The listing builds one solid part. Answer for the finished solid, in the listing's coordinates (mm). Coordinates: 2 decimals unless noted, no trailing zeros. Loops run counter-clockwise (first coordinate to the right, second up) from the corner with the lowest first, then second, coordinate; pieces in that order, holes last. Notation, with made-up numbers: (10.5, 65) - (37.5, 65) arc R22 ccw to (37.5, 86) - close; hole circle Ø10 at (89, 74). An arc over 180 degrees is marked (long way). Put each result on its own line as item: value.
```python
from build123d import *

# Parameters (mm, degrees)
SKETCH1_W              = 78
SKETCH1_H              = 120
SKETCH1_R              = 1.5
SKETCH1_W_2            = 4
SKETCH1_H_2            = 68
MAIN_SLIDER_TOP_DEPTH  = 2
SLIDE_TOP_CONTOURING_R = 4


with BuildPart() as part:
    # Sketch1 → Main Slider Top (new body)
    with BuildSketch(Plane.XY):
        with Locations((39, 60)):
            Rectangle(SKETCH1_W, SKETCH1_H)
        with Locations((14, 108)):
            Circle(SKETCH1_R, mode=Mode.SUBTRACT)
        with Locations((32, 108)):
            Circle(SKETCH1_R, mode=Mode.SUBTRACT)
        with Locations((14, 24)):
            Circle(SKETCH1_R, mode=Mode.SUBTRACT)
        with Locations((32, 24)):
            Circle(SKETCH1_R, mode=Mode.SUBTRACT)
        with Locations((46, 108)):
            Circle(SKETCH1_R, mode=Mode.SUBTRACT)
        with Locations((64, 108)):
            Circle(SKETCH1_R, mode=Mode.SUBTRACT)
        with Locations((46, 24)):
            Circle(SKETCH1_R, mode=Mode.SUBTRACT)
        with Locations((64, 24)):
            Circle(SKETCH1_R, mode=Mode.SUBTRACT)
        with Locations((23, 73)):
            Rectangle(SKETCH1_W_2, SKETCH1_H_2, mode=Mode.SUBTRACT)
        with Locations((55, 73)):
            Rectangle(SKETCH1_W_2, SKETCH1_H_2, mode=Mode.SUBTRACT)
        with BuildLine():
            Line((32, 118), (32, 116))
            add(Edge.make_bspline(
                [(32, 116), (39, 116.4), (46, 116)],
                knots=[0, 0, 0, 1, 1, 1], degree=2))
            Line((46, 116), (46, 118))
            add(Edge.make_bspline(
                [(32, 118), (39, 117.6), (46, 118)],
                knots=[0, 0, 0, 1, 1, 1], degree=2))
        make_face(mode=Mode.SUBTRACT)
        with BuildLine():
            Line((46, 2), (46, 4))
            add(Edge.make_bspline(
                [(32, 4), (39, 3.6), (46, 4)],
                knots=[0, 0, 0, 1, 1, 1], degree=2))
            Line((32, 4), (32, 2))
            add(Edge.make_bspline(
                [(32, 2), (39, 2.4), (46, 2)],
                knots=[0, 0, 0, 1, 1, 1], degree=2))
        make_face(mode=Mode.SUBTRACT)
        with BuildLine():
            Line((2, 31), (4, 31))
            add(Edge.make_bspline(
                [(4, 17), (3.6, 24), (4, 31)],
                knots=[0, 0, 0, 1, 1, 1], degree=2))
            Line((4, 17), (2, 17))
            add(Edge.make_bspline(
                [(2, 17), (2.4, 24), (2, 31)],
                knots=[0, 0, 0, 1, 1, 1], degree=2))
        make_face(mode=Mode.SUBTRACT)
        with BuildLine():
            Line((76, 17), (74, 17))
            add(Edge.make_bspline(
                [(74, 17), (74.4, 24), (74, 31)],
                knots=[0, 0, 0, 1, 1, 1], degree=2))
            Line((74, 31), (76, 31))
            add(Edge.make_bspline(
                [(76, 17), (75.6, 24), (76, 31)],
                knots=[0, 0, 0, 1, 1, 1], degree=2))
        make_face(mode=Mode.SUBTRACT)
        with BuildLine():
            Line((76, 89), (74, 89))
            add(Edge.make_bspline(
                [(74, 103), (74.4, 96), (74, 89)],
                knots=[0, 0, 0, 1, 1, 1], degree=2))
            Line((74, 103), (76, 103))
            add(Edge.make_bspline(
                [(76, 103), (75.6, 96), (76, 89)],
                knots=[0, 0, 0, 1, 1, 1], degree=2))
        make_face(mode=Mode.SUBTRACT)
        with BuildLine():
            Line((2, 103), (4, 103))
            add(Edge.make_bspline(
                [(4, 103), (3.6, 96), (4, 89)],
                knots=[0, 0, 0, 1, 1, 1], degree=2))
            Line((4, 89), (2, 89))
            add(Edge.make_bspline(
                [(2, 103), (2.4, 96), (2, 89)],
                knots=[0, 0, 0, 1, 1, 1], degree=2))
        make_face(mode=Mode.SUBTRACT)
    extrude(amount=MAIN_SLIDER_TOP_DEPTH)

    # Slide Top Contouring
    slide_top_contouring_edges = [part.edges().sort_by_distance(p)[0] for p in [
        (0, 0, 1),
        (0, 120, 1),
        (78, 120, 1),
        (78, 0, 1),
    ]]
    fillet(slide_top_contouring_edges, radius=SLIDE_TOP_CONTOURING_R)


solid = part.part
```
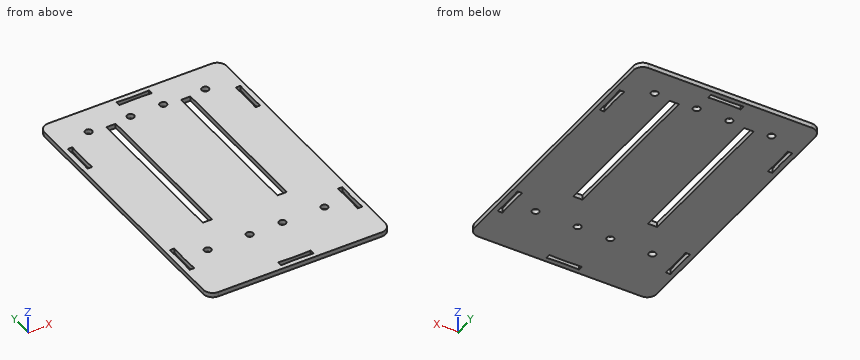
1) Each of these flat-tipped pins is pushed along its axis until it touches: pin 1 (0.6 mm diameter, centred on y = 117.5, z = 1, fed in from +X); pin 2 (0.6 mm diameter, centred on x = 3, z = 1.5, fed in from +Y); pin 3 (1 mm diameter, centred on y = 117, z = 1, fed in from -X); pin 4 (1.8 mm diameter, centred on x = 46, y = 108, fed in from +Z) (3 decimals). Where does it stop, or does it pass through?
Found:
pin 1: stops at x = 77.82
pin 2: stops at y = 119.94
pin 3: stops at x = 0.03
pin 4: passes through
2) The part is cut by section B-B (y = 44.5). Give the vertices of the cut face in (x, z), and give its area (3 significant figures).
Found:
outline: (0, 0) - (21, 0) - (21, 2) - (0, 2) - close; (25, 0) - (53, 0) - (53, 2) - (25, 2) - close; (57, 0) - (78, 0) - (78, 2) - (57, 2) - close
area: 140 mm^2
3) Straight lines are drawn through the part: L1, parallel to Y at x = 64, z = 1.55; L2, parallel to X at y = 54.5, z = 1.15; L3, parallel to Y at x = 42.5, z = 0.9. For each, find the intervals that lie inside material, in ascending order. Write a range as [from, to].
Found:
L1: y = [0, 22.5], [25.5, 106.5], [109.5, 120]
L2: x = [0, 21], [25, 53], [57, 78]
L3: y = [0, 2.15], [3.85, 116.15], [117.85, 120]
4) The part is cut by section C-C (y = 94). State how many separate pieces and enclosed holes the cut face has, and give its area (3 significant figures).
Found:
separate pieces: 5
enclosed holes: 0
area: 133 mm^2
5) The part is cut by section A-A (x = 64). Give the vertices of the cut face in (y, z), and give its area (3 significant figures).
Found:
outline: (0, 0) - (22.5, 0) - (22.5, 2) - (0, 2) - close; (25.5, 0) - (106.5, 0) - (106.5, 2) - (25.5, 2) - close; (109.5, 0) - (120, 0) - (120, 2) - (109.5, 2) - close
area: 228 mm^2
